```python
from build123d import *

# Parameters (mm, degrees)
F0_R      = 48
F1_DEPTH  = 4
F2_R      = 1
F3_R      = 35.5
F4_DEPTH  = 3.5
F5_SIZE   = 3
F6_R      = 35.5
F6_R_2    = 32.5
F7_DEPTH  = 3.5
F8_SIZE   = 2.99999
F9_R      = 60
F9_R_2    = 47.0001739343
F9_R_3    = 35.5
F10_DEPTH = 18
F11_R     = 12.5539105243
F12_R     = 3


# Not quite as in the source:
# - a fillet or chamfer is up to 0.001 mm smaller than in the source, because OpenCascade refuses the exact size


with BuildPart() as f1:
    # F0 (on Top) → F1 (new body)
    with BuildSketch(Plane.XY):
        Circle(F0_R)
    extrude(amount=F1_DEPTH)

    # F2
    f2_edges = [f1.edges().sort_by_distance(p)[0] for p in [
        (-48, 0, 4),
    ]]
    fillet(f2_edges, radius=F2_R)

    # F3 (on face) → F4 (join)
    with BuildSketch(Plane.XY.offset(4)):
        Circle(F3_R)
    extrude(amount=F4_DEPTH)

    # F5
    f5_edges = [f1.edges().sort_by_distance(p)[0] for p in [
        (-35.5, 0, 7.5),
    ]]
    chamfer(f5_edges, length=F5_SIZE)

    # F6 (on face) → F7 (join)
    with BuildSketch(Plane.XY.offset(7.5)):
        Circle(F6_R)
        Circle(F6_R_2, mode=Mode.SUBTRACT)
        Circle(F6_R_2)
    extrude(amount=F7_DEPTH)

    # F8 (size 3 in the source; OpenCascade refuses exactly that, so slightly less here)
    f8_edges = [f1.edges().sort_by_distance(p)[0] for p in [
        (-35.5, 0, 7.5),
    ]]
    chamfer(f8_edges, length=F8_SIZE)

    # F9 (on face) → F10 (join)
    with BuildSketch(Plane.XY.offset(11)):
        Circle(F9_R)
        Circle(F9_R_2, mode=Mode.SUBTRACT)
        Circle(F9_R_2)
        Circle(F9_R_3, mode=Mode.SUBTRACT)
        Circle(F9_R_3)
    extrude(amount=F10_DEPTH)

    # F11
    f11_edges = [f1.edges().sort_by_distance(p)[0] for p in [
        (-60, 0, 11),
    ]]
    fillet(f11_edges, radius=F11_R)

    # F12
    f12_edges = [f1.edges().sort_by_distance(p)[0] for p in [
        (-60, 0, 29),
    ]]
    fillet(f12_edges, radius=F12_R)


solid = f1.part
```
Input: part model. Units: mm. Frame: model coordinates. A direction names the side the tool comes from. Give positions to 0.01 mm unless a question says otherwise; leave off trailing zeros. Order: outer loops, then holes, each group sorted by start corner. A loop starts at its lowest first (then second) coordinate and runs counter-clockwise, first axis right, second up.
1. Section C-C on z = 21.75. Return the cut outline in (x, y), and give its area (3 significant figures).
Derived:
outline: circle Ø119.74 at (0, 0)
area: 11,300 mm2
2. Mould query, pull axis Z, two halves, no side actions, for faces 1 (the flat face through (7, 35, 4)), 2 (the flat face through (-1, 1, 0)), 3 (the flat face through (-1, 1, 29)). Classes: released by +Z, released by -Z, zero draft, split by the parting line, or undercut.
Derived:
face 1: undercut
face 2: released by -Z
face 3: released by +Z
3. Reachability of faces 4 (the cylindrical face through (-7.696, -34.656, 4.246)), 5 (the cylindrical face through (-47.954, 2.11, 1.479)), 6 (the cylindrical face through (-59.94, 2.64, 24.76)) from +Z, -Z, +X, -X, +Y, -Y: full face, straight path, thin tool, end or side. Return the list, or none.
Derived:
face 4: none
face 5: -Z
face 6: +Z, -Z
4. Pin query (flat end, axial travel): pin 1 (5 mm diameter, centred on x = -44.5, z = 20.5, fed in from -Y); pin 2 (3 mm diameter, centred on y = -22, z = 3.5, fed in from +X); pin 3 (1 mm diameter, centred on y = 23, z = 4, fed in from -X). Return the tip coordinate at first contact, or that it passes through.
Derived:
pin 1: stops at y = -42.44
pin 2: stops at x = 43.37
pin 3: stops at x = -42.07
5. Material intervals for L1, parallel to Z at x = 23, y = -30; L2, parallel to X at y = 18.5, z = 10; L3, parallel to Y at x = -1.5, z = 27.75, sorted ascending.
Derived:
L1: z = 0 to 4, 11 to 29
L2: x = -29.71 to 29.71
L3: y = -59.42 to 59.42
